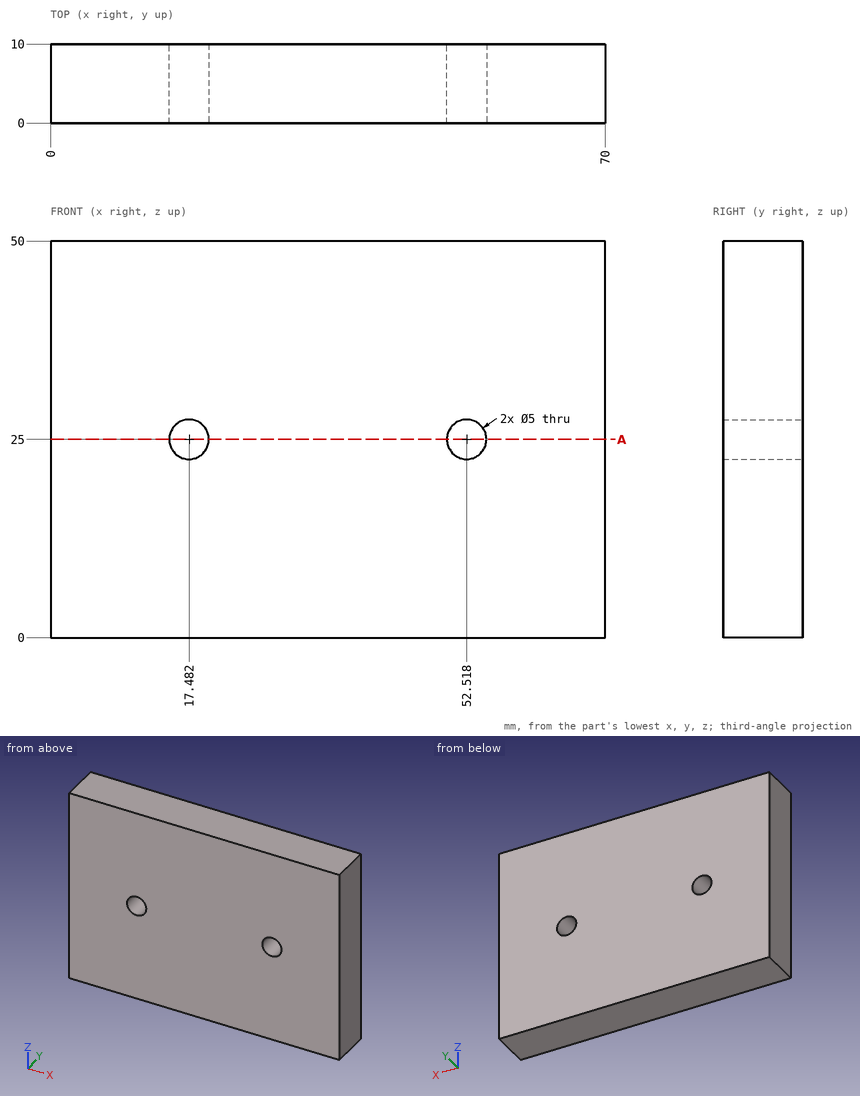
The drawing under review shows one solid part. Ordinate dimensions are in mm from its lowest x, y, z. Coordinates: 2 decimals unless noted, no trailing zeros. Order: outer loops, then holes, each group sorted by start corner. A loop starts at its lowest first (then second) coordinate and runs counter-clockwise, first axis right, second up. Notation, with made-up numbers: M 50.5,89 L 55.5,89 A19 cw 55.5,98 Z; hole C -22.75,62.25 d6. An arc over 180 degrees is marked long. Use a Markdown table: item, result.
(1) Wall thickness on probe 1 along X at (y, z) = (2, 25.5); probe 2 along Z at (x, y) = (19.5, 2.75) (1 decimal): over which ranges is each line inside the solid? List them lowest first.
Worked answers:
| item | result |
|---|---|
| probe 1 | x = 0 to 15.03, 19.93 to 50.07, 54.97 to 70 |
| probe 2 | z = 0 to 23.5, 26.5 to 50 |
(2) For P1, Ø6, axis at x = 17.48, z = 25, coming from the -Y side; P2, Ø4, axis at x = 52.52, z = 25, coming from the -Y side, all flat-tipped, find the tip position at first contact; note any pin that passes through.
Worked answers:
| item | result |
|---|---|
| P1 | stops at y = 0 |
| P2 | passes through |
(3) Add section A-A (z = 25). Give the boundary of the cut face in (x, y), then the cut area to 3 significant figures.
Worked answers:
| item | result |
|---|---|
| outline | M 0,0 L 14.98,0 L 14.98,10 L 0,10 Z; M 19.98,0 L 50.02,0 L 50.02,10 L 19.98,10 Z; M 55.02,0 L 70,0 L 70,10 L 55.02,10 Z |
| area | 600 mm2 |
